Geometry: final body of the model. Coordinates: model frame, mm. Coordinates: 2 decimals unless noted, no trailing zeros. Loops run counter-clockwise (first coordinate to the right, second up) from the corner with the lowest first, then second, coordinate; pieces in that order, holes last. Notation, with made-up numbers: (40, 31.5) - (81, 31.5) arc R31 cw to (81, 64.5) - close; hole circle Ø6 at (71, 82). An arc over 180 degrees is marked (long way). Put each result on its own line as item: value. Start each with the question number.
1) Section B-B on z = 0.35. Output: boundary loops of the cut face in (x, y).
2) Draft query along X for faces 1 (the flat face through (-586.022, -49.3, 0.246)), 2 (the flat face through (-289, -30, 1)), 3 (the cylindrical face through (-450.46, -452, 0.51)), 4 (the cylindrical face through (-450.46, -22, 0.51)). Return one class per face: +X half, -X half, draft (parallel to the pull), parting line (faces both ways), or undercut.
3) Contact query for a flat-ended pin moving along its axis: pin 1 Ø4 at (x, y) = (-483, -395.5) entering from +Z. Output: stop coordinate, or through.
4) Section A-A on x = -460. Output: boundary loops of the cut face in (y, z).
5) Section C-C on y = -455. Output: boundary loops of the cut face in (x, z) (3 decimals), and give its area (3 significant figures).
6) Section D-D on x = -80. Output: boundary loops of the cut face in (y, z), and give its area (3 significant figures).
7) Material intervals for line 1 along Y through (x, z) = (-460, 0.8); line 2 along Y through (x, z) = (-110, 0.4); line 3 along Y through (x, z) = (-490.5, 0.8), sorted ascending. Write a range as from..to.
```python
from build123d import *

# Parameters (mm, degrees)
F1_DEPTH = 0.5
F3_DEPTH = 0.5
F4_R     = 10
F5_DEPTH = 1.001


with BuildPart() as f1:
    # F0 (on Top) → F1 (new body)
    with BuildSketch(Plane.XY):
        Polygon((0, 0), (-570, 0), (-602.5, -100), (-527.5, -480), (-42.5, -480), (32.5, -100), align=None)
    extrude(amount=F1_DEPTH)

    # F2 (on face) → F3 (join)
    with BuildSketch(Plane.XY.offset(0.5)):
        Polygon((0, 0), (-570, 0), (-520, -60), (-50, -60), align=None)
        Polygon((-527.5, -480), (-42.5, -480), (-50, -420), (-520, -420), align=None)
    extrude(amount=F3_DEPTH)

    # F4 (on face) → F5 (cut, through all)
    with BuildSketch(Plane.XY.offset(1)):
        with Locations((-460, -25)):
            Circle(F4_R)
        with Locations((-460, -455)):
            Circle(F4_R)
        with Locations((-110, -25)):
            Circle(F4_R)
        with Locations((-110, -455)):
            Circle(F4_R)
    extrude(amount=-F5_DEPTH, mode=Mode.SUBTRACT)


solid = f1.part
```
Answer block:
1. outline: (-602.5, -100) - (-527.5, -480) - (-42.5, -480) - (32.5, -100) - (0, 0) - (-570, 0) - close; hole circle Ø20 at (-460, -455); hole circle Ø20 at (-460, -25); hole circle Ø20 at (-110, -455); hole circle Ø20 at (-110, -25)
2. face 1: -X half
2. face 2: draft
2. face 3: undercut
2. face 4: undercut
3. pin 1: stops at z = 0.5
4. outline: (-480, 0) - (-465, 0) - (-465, 1) - (-480, 1) - close; (-445, 0) - (-35, 0) - (-35, 1) - (-60, 1) - (-60, 0.5) - (-420, 0.5) - (-420, 1) - (-445, 1) - close; (-15, 0) - (0, 0) - (0, 1) - (-15, 1) - close
5. outline: (-532.434, 0) - (-470, 0) - (-470, 1) - (-524.375, 1) - (-524.375, 0.5) - (-532.434, 0.5) - close; (-450, 0) - (-120, 0) - (-120, 1) - (-450, 1) - close; (-100, 0) - (-37.566, 0) - (-37.566, 0.5) - (-45.625, 0.5) - (-45.625, 1) - (-100, 1) - close
5. area: 447 mm²
6. outline: (-480, 0) - (0, 0) - (0, 1) - (-60, 1) - (-60, 0.5) - (-420, 0.5) - (-420, 1) - (-480, 1) - close
6. area: 300 mm²
7. line 1: y = -480..-465, -445..-420, -60..-35, -15..0
7. line 2: y = -480..-465, -445..-35, -15..0
7. line 3: y = -480..-420, -60..0
